Input: part model. Units: mm. Frame: model coordinates. A direction names the side the tool comes from. Give positions to 0.01 mm unless a question says otherwise; leave off trailing zeros. Write each loop counter-clockwise with the first axis right and the second up, starting at its lowest first coordinate (ties: lowest second). Pieces come first, ordered by that corner, then holes. Notation, with made-up numbers: (4, 81.25) - (14, 81.25) arc R26 cw to (14, 100.25) - close; hole circle Ø9 at (58.25, -13.75). An arc over 180 degrees is marked (long way). Answer as a JSON object with one key per item and string values. Group by question number.
Autodesk Inventor part; units mm, degrees
ref_plane "YZ Plane" through (0, 0, 0) normal (1, 0, 0) x (0, 1, 0)
ref_plane "XZ Plane" through (0, 0, 0) normal (0, 1, 0) x (-1, 0, 0)
ref_plane "XY Plane" through (0, 0, 0) normal (0, 0, 1) x (1, 0, 0)
sketch "スケッチ1" plane through (0, 0, 0) normal (0, 0, 1) x (1, 0, 0)
  line L0 (-6, -2.75) -> (6, -2.75)
  line L1 (6, -2.75) -> (6, 2.75)
  line L2 (6, 2.75) -> (-6, 2.75)
  line L3 (-6, 2.75) -> (-6, -2.75)
  line L4 (-6, -2.75) -> (6, 2.75) construction
  line L5 (6, -2.75) -> (-6, 2.75) construction
  point P0 (0, 0)
  point P1 (0, 0)
  point P2 (0, 0)
  dimension "d0" = 12
  dimension "d1" = 5.5
extrude "押し出し1" add sketch "スケッチ1" along normal mid plane 1
sketch "スケッチ2" plane through (-6, 2.75, 0.5) normal (0, 1, 0) x (1, 0, 0)
  circle A0 centre (14, 1.75) radius 1.75
  line L0 (12, 0) -> (0, 0)
  line L1 (12, 1) -> (12, 0)
  circle A1 centre (14, 1.75) radius 2
  line L2 (12, 0) -> (13.7345, -0.2323)
  line L3 (12, 1) -> (12, 1.75)
  point P0 (6, 0.5)
  dimension "d4" = 3.5
  dimension "d5" = 4
extrude "押し出し2" add sketch "スケッチ2" against normal blind 0.5 contours A0 | L3 A1 L2 L1 | A1
sketch "スケッチ3" plane through (-6, 2.75, 0.5) normal (0, 1, 0) x (1, 0, 0)
  arc A0 (13.7345, -0.2323) -> (12, 1.75) centre (14, 1.75) ccw
  circle A1 centre (14, 1.75) radius 1.75
  point P0 (6, 0.5)
  dimension "d8" = 3.5
extrude "押し出し3" add sketch "スケッチ3" along normal blind 1.5
sketch "スケッチ4" plane through (8, 4.25, -1.25) normal (0, 1, 0) x (1, 0, 0)
  circle A0 centre (0, 0) radius 1.25
  circle A1 centre (0, 0) radius 1.75
  point P0 (-8, -1.25)
  dimension "d11" = 2.5
extrude "押し出し4" add sketch "スケッチ4" along normal blind 3 contours A0
sketch "スケッチ5" plane through (0, 0, 0.5) normal (0, 0, 1) x (1, 0, 0)
  line L0 (-6, 2.75) -> (-6, -2.75)
  line L1 (6, -2.75) -> (6, 2.25)
  line L2 (-6, 0) -> (6, 0) construction
  point P0 (0, 0)
  point P1 (-4, 0)
  point P2 (4, 0)
  point P3 (0, 0)
  dimension "d14" = 4
  dimension "d15" = 4
hole "穴1" at (-4, 0, 0.5) at (4, 0, 0.5) direction (0, 0, -1) diameter 2.1 depth 4 tip angle 118
fillet "フィレット1" radius 1 3 edges at (6, -2.75, 0) (-6, -2.75, 0) (-6, 2.75, 0)
properties part number "hinge"
1) Reachability of faces 4 (the face through (6.75, 5.73, -1.2)), 5 (the face through (0, 0, 0.5)), 6 (the face through (8, 2.25, -1)) from +Z, -Z, +X, -X, +Y, -Y: full face, straight path, thin tool, end or side. Return the list, or none.
2) Cut plane A-A on x = 4. Return the cut outline in (y, z), and give its area (3 significant figures).
3) Pin query (flat end, axial travel): P1, Ø0.8, axis at y = -0.5, z = 0, coming from the +X side; P2, Ø1, axis at x = -1, y = 5, coming from the +Z side; P3, Ø1.6, axis at x = -0.5, y = 0, coming from the +Z side; P4, Ø3, axis at x = 1.5, y = -0.5, coming from the -Z side. Return the tip coordinate at first contact, or that it passes through.
4) Cut plane C-C on z = -1.85. Return the cut outline in (x, y).
5) Mould query, pull axis X, two halves, no side actions, for faces 1 (the face through (-5.04, 0.14, -0.01)), 2 (the face through (3, 2.75, 0)), 3 (the face through (6, 0, 0)). Classes: +X half, -X half, draft (parallel to the pull), parting line (faces both ways), or undercut.
6) Cut plane B-B on x = 8. Return the cut outline in (y, z).
7) Line query: line 1 along X through (y, z) = (0, 0); line 2 along Y through (x, z) = (-4, -0.3); line 3 along Z through (x, y) = (-3.75, -1.25). Output: solid intervals per line, ascending. Write a range as from..to.
8) Cut plane D-D on y = 4. Return the cut outline in (x, z).
Filled in:
{
 "1": {"face 4": "+Y", "face 5": "+Z, -X, +Y, -Y", "face 6": "+Z, -Z, +X, -Y"},
 "2": {"outline": "(-2.75, -0.5) - (-1.05, -0.5) - (-1.05, 0.5) - (-2.75, 0.5) - close; (1.05, -0.5) - (2.75, -0.5) - (2.75, 0.5) - (1.05, 0.5) - close", "area": "3.40 mm²"},
 "3": {"P1": "stops at x = 6", "P2": "passes through", "P3": "stops at z = 0.5", "P4": "stops at z = -0.5"},
 "4": {"outline": "(6.09, 2.25) - (9.91, 2.25) - (9.91, 2.75) - (9.64, 2.75) - (9.64, 4.25) - (9.1, 4.25) - (9.1, 7.25) - (6.9, 7.25) - (6.9, 4.25) - (6.36, 4.25) - (6.36, 2.75) - (6.09, 2.75) - close"},
 "5": {"face 1": "undercut", "face 2": "draft", "face 3": "+X half"},
 "6": {"outline": "(2.25, -3.25) - (2.75, -3.25) - (2.75, -3) - (4.25, -3) - (4.25, -2.5) - (7.25, -2.5) - (7.25, 0) - (4.25, 0) - (4.25, 0.5) - (2.75, 0.5) - (2.75, 0.75) - (2.25, 0.75) - close"},
 "7": {"line 1": "x = -6..-5.05, -2.95..2.95, 5.05..6", "line 2": "y = -2.75..-1.05, 1.05..2.75", "line 3": "z = -0.5..0.5"},
 "8": {"outline": "circle Ø3.5 at (8, -1.25)"}
}
